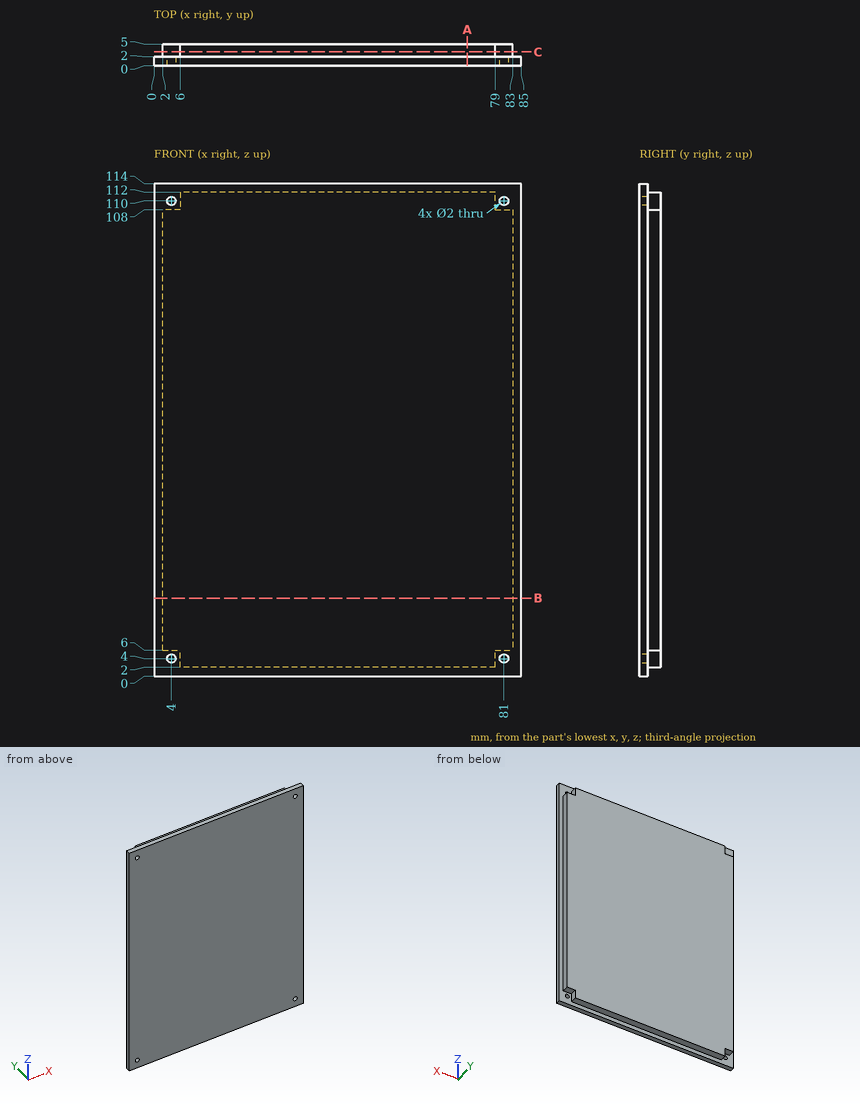
Here's the drawing with two shaded views (mm, measured from the low corner). I have some questions. Coordinates: 2 decimals unless noted, no trailing zeros. Loops run counter-clockwise (first coordinate to the right, second up) from the corner with the lowest first, then second, coordinate; pieces in that order, holes last. Notation, with made-up numbers: M 75.25,28.25 L 99.25,28.25 A35 ccw 99.25,62.25 Z; hole C 5.5,1 d5. An arc over 180 degrees is marked long. Return JSON: item names as keys, results as strings. Group by question number.
Item 1: If I drill on L1, parallel to X at y = 0.6, z = 110; L2, parallel to Z at x = 4, y = 1; L3, parallel to Z at x = 81.5, y = 1.9, over which ranges is the centre line in solid material (lowest first)? Write a range as from..to.
Item 2: Imagine slicing it at C-C (y = 3.2). Please give me the cut outline in (x, z).
Item 3: Imagine slicing it at B-B (z = 18). Please give me the cut outline in (x, y).
Item 4: I'm going to push flat-ended pins straight in: pin 1 Ø2.5 at (x, y) = (58.5, 3.5) entering from +Z; pin 2 Ø2.5 at (y, z) = (3, 33) entering from +X; pin 3 Ø3 at (x, z) = (81, 110) entering from +Y; pin 4 Ø0.9 at (x, y) = (51.5, 3.5) entering from -Z. Where does each tip first touch, or does it pass through?
Item 5: Imagine slicing it at A-A (x = 72.5). Please give me the cut outline in (y, z), and give its area (3 significant figures).
Verdict:
{
 "1": {"L1": "x = 0..3, 5..80, 82..85", "L2": "z = 0..3, 5..109, 111..114", "L3": "z = 0..3.13, 4.87..109.13, 110.87..114"},
 "2": {"outline": "M 2,6 L 6,6 L 6,2 L 79,2 L 79,6 L 83,6 L 83,108 L 79,108 L 79,112 L 6,112 L 6,108 L 2,108 Z"},
 "3": {"outline": "M 0,0 L 85,0 L 85,2 L 83,2 L 83,5 L 2,5 L 2,2 L 0,2 Z"},
 "4": {"pin 1": "stops at z = 112", "pin 2": "stops at x = 85", "pin 3": "stops at y = 2", "pin 4": "stops at z = 2"},
 "5": {"outline": "M 0,0 L 2,0 L 2,2 L 5,2 L 5,112 L 2,112 L 2,114 L 0,114 Z", "area": "558 mm^2"}
}
